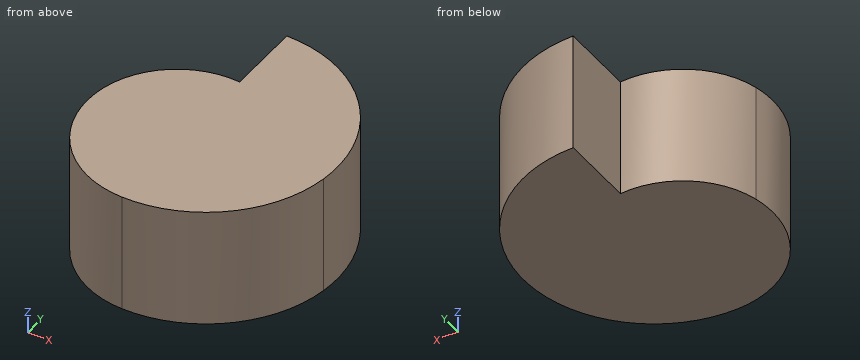
Autodesk Inventor part; units mm, degrees
ref_plane "YZ Plane" through (0, 0, 0) normal (1, 0, 0) x (0, 1, 0)
ref_plane "XZ Plane" through (0, 0, 0) normal (0, 1, 0) x (-1, 0, 0)
ref_plane "XY Plane" through (0, 0, 0) normal (0, 0, 1) x (1, 0, 0)
sketch "Sketch2" plane through (0, 0, 0) normal (0, 0, 1) x (1, 0, 0)
  circle A0 centre (0, 0) radius 5 construction
  circle A1 centre (0, 0) radius 2.5 construction
  circle A2 centre (0, 0) radius 3.125 construction
  circle A3 centre (0, 0) radius 3.75 construction
  circle A4 centre (0, 0) radius 4.375 construction
  arc A5 (4.375, 0) -> (-0.0123, 5) centre (0.032, 0.6141) ccw
  arc A6 (0, -3.75) -> (4.375, 0) centre (0.0571, 0.6105) ccw
  arc A7 (-3.1163, 0.2327) -> (0, -3.75) centre (0.0424, -0.5062) ccw
  arc A8 (-0.0123, 2.5) -> (-3.1163, 0.2327) centre (-0.2458, -0.4388) ccw
  line L0 (-0.0123, 5) -> (-0.0123, 2.5)
  dimension "d6" = 5
  dimension "d7" = 2.5
  dimension "d9" = 0.625
  dimension "d10" = 1.25
  dimension "d11" = 1.875
extrude "Extrusion1" add sketch "Sketch2" along normal blind 4
properties part number "Snail Cam"
Work out the finished part from the listing and answer in its coordinate system (mm). Round coordinates to 2 decimals unless told otherwise and drop trailing zeros. Order: outer loops, then holes, each group sorted by start corner. A loop starts at its lowest first (then second) coordinate and runs counter-clockwise, first axis right, second up. Notation, with made-up numbers: M 17.25,19 L 72.25,19 A19 ccw 72.25,48 Z; hole C 41.25,-1.5 d11. An arc over 180 degrees is marked long. One line per item, written item: value.
Q1. Flat-ended cylindrical pins translate along their axes: pin 1 (1.5 mm diameter, centred on x = -1.5, z = 3, fed in from -Y); pin 2 (2 mm diameter, centred on x = 1.5, z = 1, fed in from +Y). Find the tip coordinate at first contact, or state that the pin passes through.
Derived:
pin 1: y = -3.65
pin 2: y = 4.98
Q2. Find section C-C on x = -1.25. Write down the section's boundary in (y, z).
Derived:
outline: M -3.48,0 L 2.33,0 L 2.33,4 L -3.48,4 Z
Q3. Find section B-B on y = -0.5. Write down the section's boundary in (x, z).
Derived:
outline: M -3.2,0 L 4.27,0 L 4.27,4 L -3.2,4 Z
Q4. Find section A-A on z = 2.6. Write down the section's boundary in (x, y) (3 decimals), then the cut area to 3 significant figures.
Derived:
outline: M -3.116,0.233 A3.244 ccw 0,-3.75 A4.361 ccw 4.375,0 A4.386 ccw -0.012,5 L -0.012,2.5 A2.948 ccw Z
area: 46.4 mm²
Q5. Straight lines are drawn through the part: line 1 (Y direction, x = -2.25, z = 1.8); line 2 (Y direction, x = 4, z = 1.75); line 3 (X direction, y = 4.25, z = 0.25). For each, find the intervals that lie inside material, in ascending order.
Derived:
line 1: -2.8 to 1.72
line 2: -1.25 to 2.48
line 3: -0.01 to 2.49
